Input: part model. Units: mm. Frame: model coordinates. A direction names the side the tool comes from. Coordinates: 2 decimals unless noted, no trailing zeros. Write each loop counter-clockwise with the first axis right and the second up, starting at its lowest first coordinate (ties: lowest second). Pieces come first, ordered by that corner, then holes. Notation, with made-up numbers: (27, 26.25) - (41, 26.25) arc R16 ccw to (41, 44.25) - close; hole circle Ø11 at (32.5, 36.5). An arc over 180 degrees is marked (long way). Use a Markdown table: item, result. Add a question column.
Q1. Section query B-B (z = 1). Return the cut outline in (x, y), then the cut area to 3 significant figures.
Q2. Pin query (flat end, axial travel): P1, Ø1.3, axis at x = 0.5, z = 14.5, coming from the +Y side; P2, Ø0.5, axis at y = 10, z = 11.5, coming from the -X side; P3, Ø2, axis at y = -1, z = 15, coming from the -X side. Return the tip coordinate at first contact, or that it passes through.
Q3. Mould query, pull axis Z, two halves, no side actions, for faces 6 (the face through (-0.58, 0.91, -0.83)), 7 (the face through (0, 1, 1.25)), 8 (the face through (0, 9, 14)). Classes: released by +Z, released by -Z, zero draft, split by the parting line, or undercut.
Q4. Material intervals for probe 1 along Y at (x, z) = (-6.25, 12); probe 2 along Z at (x, y) = (-2.25, 3.5); probe 3 along Y at (x, z) = (1.5, 6.5), sorted ascending. Write a range as from..to.
Q5. Section query A-A (y = 5.75). Return the cut outline in (x, z).
Q6. Section query C-C (x = -1.5). Return the cut outline in (y, z).
Q7. Set-up query: faces 1 (the face through (0.03, 6.97, 1.66)), 2 (the face through (-2.5, -2, 15)), 3 (the face through (-0.58, 0.91, 16.03)), 4 (the face through (0, -1.8, -1)), 5 (the face through (-6, 12.3, 11)). Return all of +Z, -Z, +X, -X, +Y, -Y with unobstructed straight access to the full face (end or side cutting, diameter ignored); none if empty.
Q8. Section query D-D (y = 8.75). Return the cut outline in (x, z), then the cut area to 3 significant figures.
from build123d import *

# Parameters (mm, degrees)
PAD017_DEPTH              = 5
PAD020_DEPTH              = 6.25
SKETCH038_W               = 10
SKETCH038_H               = 1.65
PAD021_DEPTH              = 5
SKETCH078_W               = 12.5
SKETCH078_H               = 1.65
PAD047_DEPTH              = 10
SKETCH076_W               = 9.6
SKETCH076_H               = 1.65
PAD048_DEPTH              = 10
SKETCH075_W               = 12.5
SKETCH075_H               = 1.65
PAD049_DEPTH              = 7.1
SKETCH077_W               = 12.5
SKETCH077_H               = 1.65
PAD050_DEPTH              = 10
LINEARPATTERN017_COUNT    = 2
LINEARPATTERN017_PITCH    = 3.3
CHAMFER007_SIZE           = 1
MIRROR009_PLACEMENT_ANGLE = 90


with BuildPart() as obj1:
    # Sketch034 → Pad017 (new body)
    with BuildSketch(Plane.XY):
        with BuildLine():
            Line((-1.35, -1.8), (-1.35, 6))
            ThreePointArc((0, 7.35), (-0.954594, 6.954594), (-1.35, 6))
            Line((0, 9), (0, 7.35))
            Line((-2.6, 9), (0, 9))
            Line((-2.6, -1.8), (-2.6, 9))
            Line((-3.85, -1.8), (-2.6, -1.8))
            ThreePointArc((-3.85, -1.8), (-3.439949, -2.789949), (-2.45, -3.2))
            Line((-1.35, -3.2), (-2.45, -3.2))
            Line((-1.35, -1.8), (-1.35, -3.2))
        make_face()
    extrude(amount=PAD017_DEPTH)

    # Sketch037 → Pad020 (join)
    with BuildSketch(Plane.XY):
        Polygon((-1.35, 0.2), (-1.35, 1.6), (-2.6, 1.6), (-3.85, 1.6), (-3, 0.2), (-2.6, 0.2), align=None)
    extrude(amount=PAD020_DEPTH)


with BuildPart() as body026:
    # Mirror002: instance of _obj1
    add(obj1.part.mirror(Plane(origin=(5, 0, 0), x_dir=(0, 1, 0), z_dir=(-1, 0, 0))))

    # Fusion002: union _obj1
    add(obj1.part)


with BuildPart() as body026_1:
    # Clone003 placement: moved
    add(body026.part.moved(Location((-5, 0, 0))))

    # Sketch038 → Pad021 (new body)
    with BuildSketch(Plane.XY):
        with Locations((0, 8.175)):
            Rectangle(SKETCH038_W, SKETCH038_H)
    extrude(amount=PAD021_DEPTH)

    # Sketch078 → Pad047 (new body)
    with BuildSketch(Plane.XY):
        with Locations((1.35, 8.175)):
            Rectangle(SKETCH078_W, SKETCH078_H)
    extrude(amount=PAD047_DEPTH)

    # Sketch076 → Pad048 (join)
    with BuildSketch(Plane.XY):
        with Locations((2.8, 9.825)):
            Rectangle(SKETCH076_W, SKETCH076_H)
    pad048 = extrude(amount=PAD048_DEPTH)

    # Sketch075 → Pad049 (join)
    with BuildSketch(Plane.XY):
        with Locations((1.35, 9.825)):
            Rectangle(SKETCH075_W, SKETCH075_H)
    pad049 = extrude(amount=PAD049_DEPTH)

    # Sketch077 → Pad050 (join)
    with BuildSketch(Plane.XY):
        with Locations((1.35, 11.475)):
            Rectangle(SKETCH077_W, SKETCH077_H)
    pad050 = extrude(amount=PAD050_DEPTH)

    # LinearPattern017: Pad050, Pad049, Pad048 ×2
    with Locations(*[(0, i * LINEARPATTERN017_PITCH, 0) for i in range(1, LINEARPATTERN017_COUNT)]):
        add(pad050)
        add(pad049)
        add(pad048)

    # Chamfer007
    chamfer007_edges = [body026_1.edges().sort_by_distance(p)[0] for p in [
        (-4.9, 8.175, 10),
        (-4.9, 11.475, 10),
        (-4.9, 14.775, 10),
    ]]
    chamfer(chamfer007_edges, length=CHAMFER007_SIZE)


with BuildPart() as mirror009:
    # Mirror009: instance of Body026
    add(body026_1.part.mirror(Plane(origin=(0, 0, 0), x_dir=(0, -1, 0), z_dir=(1, 0, 0))))


with BuildPart() as mirror009_1:
    # Mirror009 placement: moved
    add(mirror009.part.moved(Location((2.5, 0, 7.6))).rotate(Axis((2.5, 0, 7.6), (0, -1, 0)), MIRROR009_PLACEMENT_ANGLE))


solid = mirror009_1.part
Values follow:
| question | item | result |
|---|---|---|
| 1 | outline | (-7.5, 7.35) - (-2.5, 7.35) - (-2.5, 1.6) - (-3.75, 1.6) - (-3.75, 0.2) - (-2.5, 0.2) - (-2.5, -3.2) - (2.5, -3.2) - (2.5, 15.6) - (-7.5, 15.6) - close |
| 1 | area | 137 mm2 |
| 2 | P1 | y = 9 |
| 2 | P2 | x = -4.6 |
| 2 | P3 | x = -2.5 |
| 3 | face 6 | released by -Z |
| 3 | face 7 | undercut |
| 3 | face 8 | zero draft |
| 4 | probe 1 | 7.35..9, 10.65..12.3, 13.95..15.6 |
| 4 | probe 2 | 0..1.25, 13.95..15.2 |
| 4 | probe 3 | 7.35..15.6 |
| 5 | outline | (-2.5, 0) - (2.5, 0) - (2.5, 1.25) - (-2.5, 1.25) - close; (-2.5, 13.95) - (2.5, 13.95) - (2.5, 15.2) - (-2.5, 15.2) - close |
| 6 | outline | (-3.2, 0.15) arc R1.4 ccw to (-1.8, -1.25) - (-1.8, 0) - (0.2, 0) - (0.2, -0.4) - (1.6, -1.25) - (1.6, 0) - (15.6, 0) - (15.6, 12.5) - (9, 12.5) - (9, 15.2) - (1.6, 15.2) - (1.6, 16.45) - (0.2, 15.6) - (0.2, 15.2) - (-1.8, 15.2) - (-1.8, 16.45) arc R1.4 ccw to (-3.2, 15.05) - (-3.2, 13.95) - (6, 13.95) arc R1.35 cw to (7.35, 12.6) - (7.35, 2.6) arc R1.35 cw to (6, 1.25) - (-3.2, 1.25) - close |
| 7 | face 1 | +X, -X, -Y |
| 7 | face 2 | +Z, -Z, -X, -Y |
| 7 | face 3 | +Z, +X, -X |
| 7 | face 4 | -Z, +X, -X |
| 7 | face 5 | +Z, -X |
| 8 | outline | (-7.5, 0) - (2.5, 0) - (2.5, 15.2) - (-2.5, 15.2) - (-2.5, 12.5) - (-6.5, 12.5) - (-7.5, 11.5) - close |
| 8 | area | 138 mm2 |
